Part model, mm, in its own coordinate system. Round coordinates to 2 decimals unless told otherwise and drop trailing zeros. Loops run counter-clockwise (first coordinate to the right, second up) from the corner with the lowest first, then second, coordinate; pieces in that order, holes last. Notation, with made-up numbers: M -35,73.25 L 16,73.25 A33 ccw 16,103.25 Z; hole C 19.25,31.25 d8. An arc over 180 degrees is marked long. Answer as CSV lines item,"result". Start each with the question number.
Item 1: Band-saw the part on A-A (z = 36). Give the cut face in (x, y).
Item 2: Band-saw the part on C-C (y = 2.6). Give the cut face in (x, z).
Item 3: Wall check: line 1 (Z direction, x = 0, y = 3.75); line 2 (Z direction, x = -2, y = 1.4). Give the ranges that are in metal, low to high.
Item 4: Band-saw the part on B-B (x = 0). Give the cut face in (y, z), and give its area (3 significant figures).
Item 5: Drop a flat-ended pin along its axis: pin 1 Ø1.5 at (x, z) = (-3, 78) entering from -Y. Give the stop position or say it passes through.
```python
from build123d import *

# Parameters (mm, degrees)
F0_R     = 3.5
F1_DEPTH = 6
F2_W     = 7
F2_H     = 150
F3_DEPTH = 25


with BuildPart() as f1:
    # F0 (on Front) → F1 (new body)
    with BuildSketch(Plane.XZ):
        with BuildLine():
            Line((-10, 150), (-10, 0))
            ThreePointArc((-10, 0), (0, -10), (10, 0))
            Line((10, 0), (10, 150))
            Line((10, 150), (-10, 150))
        make_face()
        Circle(F0_R, mode=Mode.SUBTRACT)
    extrude(amount=-F1_DEPTH)

    # F2 (on face) → F3 (cut)
    with BuildSketch(Plane.XZ):
        with Locations((0, 85)):
            Rectangle(F2_W, F2_H)
    extrude(amount=-F3_DEPTH, mode=Mode.SUBTRACT)


solid = f1.part
```
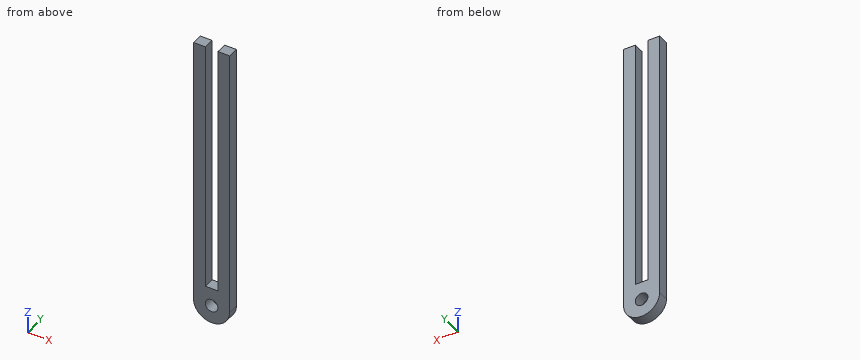
Answer block:
1,outline,"M -10,0 L -3.5,0 L -3.5,6 L -10,6 Z; M 3.5,0 L 10,0 L 10,6 L 3.5,6 Z"
2,outline,"M -10,0 A10 ccw 10,0 L 10,150 L 3.5,150 L 3.5,10 L -3.5,10 L -3.5,150 L -10,150 Z; hole C 0,0 d7"
3,line 1,"z = -10 to -3.5, 3.5 to 10"
3,line 2,"z = -9.8 to -2.87, 2.87 to 10"
4,outline,"M 0,-10 L 6,-10 L 6,-3.5 L 0,-3.5 Z; M 0,3.5 L 6,3.5 L 6,10 L 0,10 Z"
4,area,"78.0 mm^2"
5,pin 1,"stops at y = 0"
